Here's how the part is built. I have some questions about the finished solid (model axes, mm). Face numbers are marked on the shaded views. A direction names the side the tool comes from. Give positions to 0.01 mm unless a question says otherwise; leave off trailing zeros. Loops run counter-clockwise (first coordinate to the right, second up) from the corner with the lowest first, then second, coordinate; pieces in that order, holes last. Notation, with made-up numbers: M -34,12 L -24,12 A28 ccw -24,42 Z; hole C -14.75,21 d2. An arc over 180 degrees is marked long. Write item = value, one per line. Start each with the question number.
```python
from build123d import *

# Parameters (mm, degrees)
F3_START = -7.62
F3_DEPTH = 93.981
F4_R     = 1.1938
F5_DEPTH = 12.7


with BuildPart() as f1:
    # F0 (on Front) → F1 (revolve)
    with BuildSketch(Plane.XZ):
        with BuildLine():
            Line((-101.6, 0), (-40.64, 0))
            Line((-40.64, 0), (-40.64, 3.175))
            Line((-40.64, 3.175), (0, 3.175))
            Line((0, 3.175), (0, 12.7))
            Line((0, 12.7), (-6.35, 12.7))
            Line((-6.35, 12.7), (-6.35, 9.9233625935))
            ThreePointArc((-6.35, 9.9233625935), (-7.4331158517, 7.842716401), (-9.758731164, 7.5365433367))
            Line((-9.758731164, 7.5365433367), (-23.9452117528, 12.7))
            Line((-23.9452117528, 12.7), (-99.4210244843, 12.7))
            ThreePointArc((-99.4210244843, 12.7), (-101.0513051228, 6.4427853895), (-101.6, 0))
        make_face()
    revolve(axis=Axis((-71.12, 0, 0), (1, 0, 0)))

    # F2 (on Right) → F3 (cut)
    with BuildSketch(Plane.YZ.offset(F3_START)):
        with BuildLine():
            ThreePointArc((-3.175, 13.8581385114), (-3.2583413998, 14.751147695), (-3.5054871123, 15.6133136811))
            ThreePointArc((-3.5054871123, 15.6133136811), (-8.001, 13.8581385114), (-11.768782729, 10.8424977325))
            ThreePointArc((-11.768782729, 10.8424977325), (-6.4030393387, 9.3043710903), (-3.175, 13.8581385114))
        make_face()
        with BuildLine():
            ThreePointArc((3.5054871123, 15.6133136811), (5.588, 9.6786999127), (11.768782729, 10.8424977325))
            ThreePointArc((11.768782729, 10.8424977325), (8.001, 13.8581385114), (3.5054871123, 15.6133136811))
        make_face()
        with BuildLine():
            ThreePointArc((15.2742698413, -4.7708159487), (15.8190213035, -2.413), (16.002, 0))
            ThreePointArc((16.002, 0), (15.8190213035, 2.413), (15.2742698413, 4.7708159487))
            ThreePointArc((15.2742698413, 4.7708159487), (11.176, 0), (15.2742698413, -4.7708159487))
        make_face()
        with BuildLine():
            ThreePointArc((3.5054871123, -15.6133136811), (8.001, -13.8581385114), (11.768782729, -10.8424977325))
            ThreePointArc((11.768782729, -10.8424977325), (5.588, -9.6786999127), (3.5054871123, -15.6133136811))
        make_face()
        with BuildLine():
            ThreePointArc((-11.768782729, -10.8424977325), (-8.001, -13.8581385114), (-3.5054871123, -15.6133136811))
            ThreePointArc((-3.5054871123, -15.6133136811), (-3.2583413998, -14.751147695), (-3.175, -13.8581385114))
            ThreePointArc((-3.175, -13.8581385114), (-6.4030393387, -9.3043710903), (-11.768782729, -10.8424977325))
        make_face()
        with BuildLine():
            ThreePointArc((-11.176, 0), (-12.3412417626, 3.1446979389), (-15.2742698413, 4.7708159487))
            ThreePointArc((-15.2742698413, 4.7708159487), (-16.002, 0), (-15.2742698413, -4.7708159487))
            ThreePointArc((-15.2742698413, -4.7708159487), (-12.3412417626, -3.1446979389), (-11.176, 0))
        make_face()
    extrude(amount=-F3_DEPTH, mode=Mode.SUBTRACT)

    # F4 (on Front) → F5 (cut, symmetric)
    with BuildSketch(Plane.XZ):
        with Locations((-33.274, 0)):
            Circle(F4_R)
    extrude(amount=F5_DEPTH, both=True, mode=Mode.SUBTRACT)


solid = f1.part
```
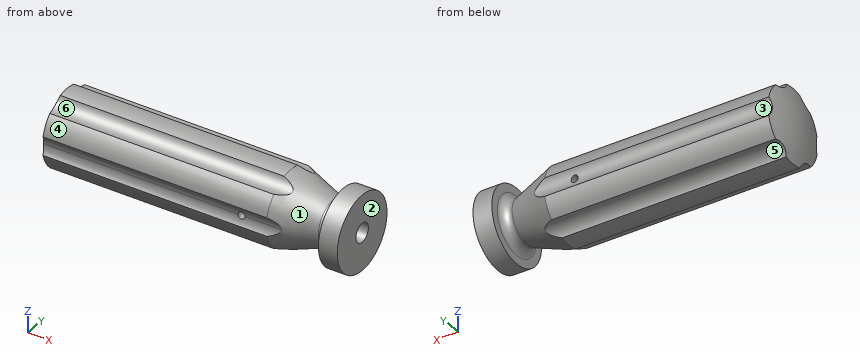
Q1. If we section it at A-A, the plane x = -83: List the corners of the cut face in (y, z) for me, then the cut area to 3 significant figures.
Q2. Will these pins go through, and if not, where does the flat tip stop? pin 1 (1.5 mm diameter, centred on y = 9, z = -6, fed in from +X); pin 2 (2 mm diameter, centred on x = -16, y = -0.5, fed in from +Z); pin 3 (12 mm diameter, centred on x = -14.5, y = -4.5, fed in from -Z); pin 4 (3 mm diameter, centred on x = -69.5, y = -9.5, fed in from +Z).
Q3. On a 3-axis mill with a long thin cutter (end or side, diameter ignored), from which of +Z, -Z, +X, -X, +Y, -Y can I reach the whole of each face in a straight line? I mean the marked faces 1 and 2. Say none if no direction works.
Q4. If we section it at B-B, the plane y = 0: List the corners of the cut face in (x, z) for me (3 decimals).
Q5. If I drill on line 1 along Z through (x, y) = (-64, 0); line 2 along Z through (x, y) = (-28.5, 0) (3 decimals); line 3 along X through (y, z) = (-4.75, 0), over which ranges is the centre line in solid material (lowest first)?
Q6. We'd pull the mould along Y, two halves only. Please class the marked faces 3, 4, 5 and 6: pulls with the +Y half, pulls with the -Y half, needs draft (parallel to the pull), parting line crosses it, or undercut.
Resolved:
q1.outline = M -12.31,-3.11 A12.7 ccw -8.85,-9.11 A4.83 cw -3.46,-12.22 A12.7 ccw 3.46,-12.22 A4.83 cw 8.85,-9.11 A12.7 ccw 12.31,-3.11 A4.83 cw 12.31,3.11 A12.7 ccw 8.85,9.11 A4.83 cw 3.46,12.22 A12.7 ccw -3.46,12.22 A4.83 cw -8.85,9.11 A12.7 ccw -12.31,3.11 A4.83 cw Z
q1.area = 468 mm²
q2.pin_1 = 0
q2.pin_2 = 10.16
q2.pin_3 = -11.07
q2.pin_4 = 9.11
q3.face_1 = none
q3.face_2 = +Z, -Z, +X, +Y, -Y
q4.outline = M -99.421,-12.7 L -23.945,-12.7 L -9.759,-7.537 A2.54 cw -6.35,-9.923 L -6.35,-12.7 L 0,-12.7 L 0,-3.175 L -40.64,-3.175 L -40.64,3.175 L 0,3.175 L 0,12.7 L -6.35,12.7 L -6.35,9.923 A2.54 cw -9.759,7.537 L -23.945,12.7 L -99.421,12.7 A38.1 ccw Z
q5.line_1 = -12.7 to 12.7
q5.line_2 = -12.7 to -3.175, 3.175 to 12.7
q5.line_3 = -101.3 to -34.47, -32.08 to 0
q6.face_3 = pulls with the +Y half
q6.face_4 = pulls with the -Y half
q6.face_5 = undercut
q6.face_6 = undercut
